from build123d import *

# Parameters (mm, degrees)
SKETCH_W        = 58
SKETCH_H        = 30
SKETCH_R        = 1.6
SKETCH_W_2      = 50.7
SKETCH_H_2      = 1.5
PAD_DEPTH       = 7
SKETCH001_W     = 19
SKETCH001_H     = 2.5
POCKET_DEPTH    = 58
POCKET001_DEPTH = 2
FILLET_R        = 3
CHAMFER_SIZE    = 0.7


with BuildPart() as part:
    # Sketch → Pad (new body)
    with BuildSketch(Plane.XY):
        Rectangle(SKETCH_W, SKETCH_H)
        with Locations((-17.186, 0)):
            Circle(SKETCH_R, mode=Mode.SUBTRACT)
        with Locations((17.186, 0)):
            Circle(SKETCH_R, mode=Mode.SUBTRACT)
        with Locations((1.15, 12.75)):
            Rectangle(SKETCH_W_2, SKETCH_H_2, mode=Mode.SUBTRACT)
        with Locations((1.15, -12.75)):
            Rectangle(SKETCH_W_2, SKETCH_H_2, mode=Mode.SUBTRACT)
    extrude(amount=PAD_DEPTH)

    # Sketch001 (on Face4 of Pad) → Pocket (cut)
    with BuildSketch(Plane(origin=(-29, 0, 0), x_dir=(0, -1, 0), z_dir=(-1, 0, 0))):
        with Locations((0, 5.75)):
            Rectangle(SKETCH001_W, SKETCH001_H)
    extrude(amount=-POCKET_DEPTH, mode=Mode.SUBTRACT)

    # Sketch002 (on Face7 of Pocket) → Pocket001 (cut)
    with BuildSketch(Plane.XY.offset(4.5)):
        Polygon((-15.569419, -2.8), (-13.952838, 0), (-15.569419, 2.8), (-18.802581, 2.8), (-20.419162, 0), (-18.802581, -2.8), align=None)
        Polygon((13.952838, 0), (15.569419, -2.8), (18.802581, -2.8), (20.419162, 0), (18.802581, 2.8), (15.569419, 2.8), align=None)
    extrude(amount=-POCKET001_DEPTH, mode=Mode.SUBTRACT)

    # Fillet
    fillet_edges = [part.edges().sort_by_distance(p)[0] for p in [
        (-29, -15, 3.5),
        (-29, 15, 3.5),
        (29, -15, 3.5),
        (29, 15, 3.5),
    ]]
    fillet(fillet_edges, radius=FILLET_R)

    # Chamfer
    chamfer_edges = [part.edges().sort_by_distance(p)[0] for p in [
        (1.15, -12, 7),
        (1.15, -13.5, 7),
        (26.5, -12.75, 7),
        (-24.2, -12.75, 7),
        (1.15, 13.5, 7),
        (1.15, 12, 7),
        (-24.2, 12.75, 7),
        (26.5, 12.75, 7),
    ]]
    chamfer(chamfer_edges, length=CHAMFER_SIZE)


solid = part.part
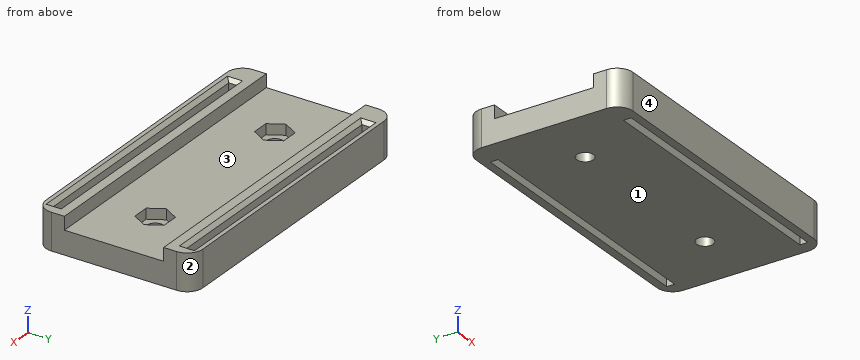
Geometry: final body of the model. Coordinates: model frame, mm. Face numbers are marked on the shaded views. Give positions to 0.01 mm unless a question says otherwise; leave off trailing zeros. Loops run counter-clockwise (first coordinate to the right, second up) from the corner with the lowest first, then second, coordinate; pieces in that order, holes last. Notation, with made-up numbers: M 42.25,82.5 L 73.25,82.5 A23 ccw 73.25,117.5 Z; hole C -17.5,-1 d1. An arc over 180 degrees is marked long. Put each result on its own line as item: value.
1) Cut plane B-B, the plane z = 3.5. Return the cut outline in (x, y).
Computed values:
outline: M -29,-12 A3 ccw -26,-15 L 26,-15 A3 ccw 29,-12 L 29,12 A3 ccw 26,15 L -26,15 A3 ccw -29,12 Z; hole M -24.2,-13.5 L 26.5,-13.5 L 26.5,-12 L -24.2,-12 Z; hole M -24.2,12 L 26.5,12 L 26.5,13.5 L -24.2,13.5 Z; hole M -20.42,0 L -18.8,-2.8 L -15.57,-2.8 L -13.95,0 L -15.57,2.8 L -18.8,2.8 Z; hole M 13.95,0 L 15.57,-2.8 L 18.8,-2.8 L 20.42,0 L 18.8,2.8 L 15.57,2.8 Z
2) First-contact query: P1, Ø2.5, axis at x = 17.186, y = 0, coming from the +Z side; P2, Ø4, axis at x = -17.186, y = 0, coming from the +Z side; P3, Ø6, axis at x = 16, y = 0.5, coming from the +Z side. Flat tips, straight axial feed; report the tip coordinate or a pass-through.
Computed values:
P1: passes through
P2: stops at z = 2.5
P3: stops at z = 4.5
3) Cut plane A-A, the plane x = -12. Return the cut outline in (y, z), plus the area to 3 significant figures.
Computed values:
outline: M -15,0 L -13.5,0 L -13.5,6.3 L -14.2,7 L -15,7 Z; M -12,0 L 12,0 L 12,6.3 L 11.3,7 L 9.5,7 L 9.5,4.5 L -9.5,4.5 L -9.5,7 L -11.3,7 L -12,6.3 Z; M 13.5,0 L 15,0 L 15,7 L 14.2,7 L 13.5,6.3 Z
area: 141 mm^2
4) Mould query, pull axis Y, two halves, no side actions, for the marked faces 1, 2, 3 and 4. Classes: released by +Y, released by -Y, zero draft, split by the parting line, or undercut.
Computed values:
face 1: zero draft
face 2: released by +Y
face 3: undercut
face 4: released by -Y
5) Material intervals for L1, parallel to Y at x = 0, z = 4.25; L2, parallel to X at y = 0, z = 1.5; L3, parallel to Y at x = -16, z = 3.5, sorted ascending. Write a range as from..to.
Computed values:
L1: y = -15..-13.5, -12..12, 13.5..15
L2: x = -29..-18.79, -15.59..15.59, 18.79..29
L3: y = -15..-13.5, -12..-2.8, 2.8..12, 13.5..15
6) Cut plane C-C, the plane y = -8.5. Return the cut outline in (x, z).
Computed values:
outline: M -29,0 L 29,0 L 29,4.5 L -29,4.5 Z
